Design review of the part built by this model. Coordinates are the model's own, in mm. A direction names the side the tool comes from. Round coordinates to 2 decimals unless told otherwise and drop trailing zeros. Loops run counter-clockwise (first coordinate to the right, second up) from the corner with the lowest first, then second, coordinate; pieces in that order, holes last. Notation, with made-up numbers: (-16.75, 29) - (33.25, 29) arc R18 ccw to (33.25, 38) - close; hole circle Ø11 at (-34.75, 67.5). An arc over 180 degrees is marked (long way). One line per question, with ' | ' between items. Start each with the question number.
from build123d import *
from build123d import SkipClean  # not in build123d's __all__

# Parameters (mm, degrees)
F0_W      = 131
F0_H      = 155.25
F0_R      = 5
F0_R_2    = 10
F1_DEPTH  = 12.7
F2_DEPTH  = 150
F3_R      = 4.7625
F4_DEPTH  = 167.951
F6_DEPTH  = 55
F9_W      = 46.4503765106
F9_H      = 23.6088857055
F10_DEPTH = 100.6187200546
F12_DEPTH = 150.001
F14_DEPTH = 89.0000760555
F15_R     = 16
F16_DEPTH = 210.4837932836
F18_W     = 28.0103459954
F18_H     = 33.3821959794
F19_DEPTH = 57.4413500726
F23_DEPTH = 37.3063087463
F25_DEPTH = 262.8513174901
F26_W     = 130
F26_H     = 33
F27_DEPTH = 25
F28_DEPTH = 47.1665114164
F29_W     = 130
F29_H     = 16.5
F30_DEPTH = 118.0664598942
F32_DEPTH = 6.5
F33_R     = 5
F34_DEPTH = 47.2060309181
F35_W     = 63.7330800295
F35_H     = 16.5
F36_DEPTH = 26
F37_W     = 33.5
F37_H     = 25
F38_DEPTH = 25
F39_R     = 5
F41_DEPTH = 150.837957859


with BuildPart() as f1:
    # F0 (on Front) → F1 (new body)
    with BuildSketch(Plane.XZ):
        with Locations((0, 77.625)):
            Rectangle(F0_W, F0_H)
        with Locations((-32.75, 57)):
            Circle(F0_R, mode=Mode.SUBTRACT)
        with Locations((32.75, 57)):
            Circle(F0_R, mode=Mode.SUBTRACT)
        with Locations((0, 89.75)):
            Circle(F0_R_2, mode=Mode.SUBTRACT)
        with Locations((-32.75, 122.5)):
            Circle(F0_R, mode=Mode.SUBTRACT)
        with Locations((32.75, 122.5)):
            Circle(F0_R, mode=Mode.SUBTRACT)
    extrude(amount=-F1_DEPTH)

    # F0 (on Front) → F2 (join)
    with BuildSketch(Plane.XZ):
        Polygon((89.5, 0), (65.5, 0), (-65.5, 0), (-65.5, -12.7), (89.5, -12.7), align=None)
    extrude(amount=-F2_DEPTH)

    # F3 (on face) → F4 (cut, through all)
    with BuildSketch(Plane(origin=(0, 0, -12.7), x_dir=(1, 0, 0), z_dir=(0, 0, -1))):
        with Locations((-40, -55.7)):
            Circle(F3_R)
        with Locations((-40, -118.2)):
            Circle(F3_R)
        with Locations((64, -118.2)):
            Circle(F3_R)
        with Locations((64, -55.7)):
            Circle(F3_R)
    extrude(amount=-F4_DEPTH, mode=Mode.SUBTRACT)

    # F5 (on face) → F6 (join)
    with BuildSketch(Plane.XZ):
        Polygon((76.5, -12.7), (-63.5, -12.7), (-44.9285714286, -100.7630571853), align=None)
    extrude(amount=-F6_DEPTH)

    # F7 (on face) → F8 (revolve)
    with BuildSketch(Plane(origin=(32.4031609217, 0, -44.6801379177), x_dir=(0.8095238095, 0, 0.5870870479), z_dir=(0.5870870479, 0, -0.8095238095))):
        Polygon((18.2698592544, -40), (54.4725659202, -40), (54.4725659202, -30), (-45.5274340798, -30), (-45.5274340798, -40), align=None)
    revolve(axis=Axis((36.0238095238, 55, -42.0543523951), (-0.8095238095, 0, -0.5870870479)))

    # F9 (on face) → F10 (cut)
    with BuildSketch(Plane.YZ.offset(89.5)):
        with Locations((57.3695674539, 11.8044428527)):
            Rectangle(F9_W, F9_H)
    extrude(amount=-F10_DEPTH, mode=Mode.SUBTRACT)

    # F11 (on Front) → F12 (cut, through all)
    with BuildSketch(Plane.XZ):
        Polygon((-55.6169226766, -72.8361010551), (-44.6262694895, -72.8361010551), (-44.6262694895, -12.6905664802), (-63.8953074813, -12.6905664802), (-63.8953074813, -72.8361010551), align=None)
        Polygon((-4.5890193433, -104.113265872), (-4.5890193433, -72.8361010551), (-44.6262694895, -72.8361010551), (-55.6169226766, -72.8361010551), (-55.6169226766, -104.113265872), align=None)
    extrude(amount=-F12_DEPTH, mode=Mode.SUBTRACT)

    # F13 (on face) → F14 (cut)
    with BuildSketch(Plane(origin=(0, 55, 0), x_dir=(-1, 0, 0), z_dir=(0, 1, 0))):
        Polygon((76.3912552581, -71.6465198879), (44.6262694895, -60.2878452083), (44.6262694895, -72.8361010551), (6.4205920826, -72.8361010551), (4.4523809524, -71.4087047902), (-10.0519139283, -91.4084170785), (37.2047263411, -125.6801223738), align=None)
        Polygon((44.6262694895, -60.2878452083), (19.1295571499, -51.1706095521), (13.2586866709, -59.2658476473), (4.4523809524, -71.4087047902), (6.4205920826, -72.8361010551), (44.6262694895, -72.8361010551), align=None)
    extrude(amount=-F14_DEPTH, mode=Mode.SUBTRACT)

    # F15 (on face) → F16 (cut, through all)
    with BuildSketch(Plane(origin=(-36.8555418741, 0, -26.7285668724), x_dir=(0, -1, 0), z_dir=(-0.8095238095, 0, -0.5870870479))):
        with Locations((-55, -55.1931115454)):
            Circle(F15_R)
        with BuildLine():
            ThreePointArc((-40, -55.1931115454), (-65.6066017178, -65.7997132632), (-55, -40.1931115454))
            Line((-55, -40.1931115454), (-55, -55.1931115454))
            Line((-55, -55.1931115454), (-40, -55.1931115454))
        make_face(mode=Mode.SUBTRACT)
        with BuildLine():
            Line((-55, -55.1931115454), (-55, -40.1931115454))
            ThreePointArc((-55, -40.1931115454), (-65.6066017178, -65.7997132632), (-40, -55.1931115454))
            Line((-40, -55.1931115454), (-55, -55.1931115454))
        make_face()
    with SkipClean():  # cleaning this boolean's faces spoils the solid; the shape is the same uncleaned
        extrude(amount=-F16_DEPTH, mode=Mode.SUBTRACT)

    # F18 (on offset) → F19 (cut)
    with BuildSketch(Plane(origin=(0, 0, -69.7121929049), x_dir=(1, 0, 0), z_dir=(0, 0, -1))):
        with Locations((-40.2482412755, -55.8588486165)):
            Rectangle(F18_W, F18_H)
    with SkipClean():  # cleaning this boolean's faces spoils the solid; the shape is the same uncleaned
        extrude(amount=-F19_DEPTH, mode=Mode.SUBTRACT)

    # F22 (on offset) → F23 (join)
    with BuildSketch(Plane(origin=(0, 66.3563400507, 0), x_dir=(-1, 0, 0), z_dir=(0, 1, 0))):
        Polygon((-19.5, -25.368578732), (9.2864632607, -47.1396760544), (25.5, -47.1396760544), (25.5, -10.8354373375), (-19.5, -10.8354373375), align=None)
    with SkipClean():  # cleaning this boolean's faces spoils the solid; the shape is the same uncleaned
        extrude(amount=-F23_DEPTH)

    # F24 (on offset) → F25 (cut, through all)
    with BuildSketch(Plane(origin=(0, 0, -107.6003174901), x_dir=(1, 0, 0), z_dir=(0, 0, -1))):
        Polygon((105.054743588, -47.2050309181), (-70.2532827854, -47.2050309181), (-70.2532827854, -164.4858419895), (108.5324063897, -164.4858419895), align=None)
    extrude(amount=-F25_DEPTH, mode=Mode.SUBTRACT)

    # F26 (on Front) → F27 (join)
    with BuildSketch(Plane.XZ):
        with Locations((0.4943662184, -6)):
            Rectangle(F26_W, F26_H)
    extrude(amount=F27_DEPTH)

    # F28 (add): a face of the model
    f28_faces = [f1.faces().sort_by_distance(p)[0] for p in [
        (-54.5656671683, 0, -17.5954279167),
    ]]
    extrude(f28_faces, amount=F28_DEPTH)

    # F29 (on face) → F30 (cut)
    with BuildSketch(Plane.XZ.offset(25)):
        Polygon((65.4943662184, -6), (102.4388783057, -6), (114.364810288, 171.1933612823), (-95.0750373681, 171.1933612823), (-95.0750373681, -6), (-64.5056337816, -6), (-64.5056337816, 10.5), (65.4943662184, 10.5), align=None)
        with Locations((0.4943662184, 2.25)):
            Rectangle(F29_W, F29_H)
    extrude(amount=-F30_DEPTH, mode=Mode.SUBTRACT)

    # F31 (on face) → F32 (cut)
    with BuildSketch(Plane.XZ):
        Polygon((-12.7527767497, -46.5), (-5.2472232503, -46.5), (-1.4944465005, -40), (-5.2472232503, -33.5), (-12.7527767497, -33.5), (-16.5055534995, -40), align=None)
    extrude(amount=-F32_DEPTH, mode=Mode.SUBTRACT)

    # F33 (on face) → F34 (cut, through all)
    with BuildSketch(Plane.XZ):
        with Locations((-9, -40)):
            Circle(F33_R)
    extrude(amount=-F34_DEPTH, mode=Mode.SUBTRACT)

    # F35 (on face) → F36 (join)
    with BuildSketch(Plane.YZ.offset(65.4943662184)):
        with Locations((6.8665400147, -14.25)):
            Rectangle(F35_W, F35_H)
    extrude(amount=F36_DEPTH)

    # F37 (on face) → F38 (join)
    with BuildSketch(Plane.XY.offset(-6)):
        with Locations((74.7443662184, -12.5)):
            Rectangle(F37_W, F37_H)
    extrude(amount=F38_DEPTH)

    # F39
    f39_edges = [f1.edges().sort_by_distance(p)[0] for p in [
        (57.994366, 0, 6.5),
        (91.494366, 0, 6.5),
        (91.494366, 19.36654, -6),
    ]]
    fillet(f39_edges, radius=F39_R)

    # F40 (on face) → F41 (cut)
    with BuildSketch(Plane(origin=(0, 0, -22.5), x_dir=(1, 0, 0), z_dir=(0, 0, -1))):
        Polygon((-64.5056337816, -47.1665114164), (-64.5056337816, 25), (-82.232825458, 25), (-82.232825458, -50.1768067479), (-64.5056337816, -50.1768067479), align=None)
    extrude(amount=-F41_DEPTH, mode=Mode.SUBTRACT)


solid = f1.part
1. Clearance check with flat-ended pins moving along their axes: P1, Ø0.7, axis at x = 83, y = 39.5, coming from the -Z side; P2, Ø1.8, axis at y = 40, z = -9, coming from the +X side; P3, Ø7.5, axis at x = 86, z = -12, coming from the +Y side; P4, Ø1.5, axis at y = -1.5, z = -64.5, coming from the -X side. State where each tip first meets the part, or that it passes through.
2. Machinability: for faces 1 (the face through (-14.6, 3.2, -36.7)), 2 (the face through (57.994, -15, 6)), 3 (the face through (89.991, 17.454, -7.426)), 4 (the face through (-49, 43, -12.691)), 5 (the face through (-44.626, 19, -42)), which of the approach directions +Z, -Z, +X, -X, +Y, -Y give a long, thin tool a straight path to every point of the face, cutting with its end or side? Answer none if there is none.
3. Take a section at A-A, the plane y = 2. Give the boundary of the cut face in (x, z).
4. The part is to be moulded in two halves that separate along Z. For faces 6 (the face through (-32.056, 18.688, -55.793)), 7 (the face through (-9, 3, -46.5)), 8 (the face through (-3.5, 0, -35.7)), say which applies: pulls with the +Z half, pulls with the -Z half, needs draft (parallel to the pull), parting line crosses it, or undercut.
5. Take a section at B-B, the plane x = -52.5. Give the boundary of the cut face in (y, z).
6. To check wall thickness, follow line 1 along Z through (x, y) = (-9, 34); line 2 along Z through (x, y) = (67, 27); line 3 along X through (y, z) = (-12, 1.5). State the ranges of each line that lie inside material, in increasing order.
Answer list:
1) P1: stops at z = -32.64 | P2: stops at x = 89.5 | P3: stops at y = 40.94 | P4: passes through
2) face 1: -Y | face 2: +Z, -X, +Y, -Y | face 3: +Z, +X, +Y | face 4: +Y | face 5: -Z, -X, +Y, -Y
3) outline: (-64.51, -22.5) - (-44.63, -22.5) - (-44.63, -60.29) - (-19.13, -51.17) - (-4.45, -71.41) - (65.49, -20.68) - (65.49, -22.5) - (91.49, -22.5) - (91.49, -11) arc R5 ccw to (86.49, -6) - (-64.51, -6) - close; hole (-16.51, -40) - (-12.75, -46.5) - (-5.25, -46.5) - (-1.49, -40) - (-5.25, -33.5) - (-12.75, -33.5) - close
4) face 6: pulls with the -Z half | face 7: undercut | face 8: needs draft
5) outline: (-25, -22.5) - (47.17, -22.5) - (47.17, -12.69) - (39.17, -12.69) - (39.17, -12.27) - (47.21, -12.27) - (47.21, -6) - (-25, -6) - close
6) line 1: z = -65.14 to -45, -35 to -6 | line 2: z = -22.5 to -6 | line 3: x = 57.99 to 91.49
